Check sheet for the drawn part. Datum: minimum x, y, z corner. Units: mm. Round coordinates to 2 decimals unless told otherwise and drop trailing zeros. Write each loop counter-clockwise with the first axis right and the second up, starting at its lowest first coordinate (ties: lowest second). Pieces come first, ordered by that corner, then holes. Notation, with made-up numbers: (79, 30) - (84, 30) arc R20 cw to (84, 62) - close; hole circle Ø5 at (38, 71.25). An arc over 180 degrees is marked (long way). Answer as a JSON object with one key per item and string values.
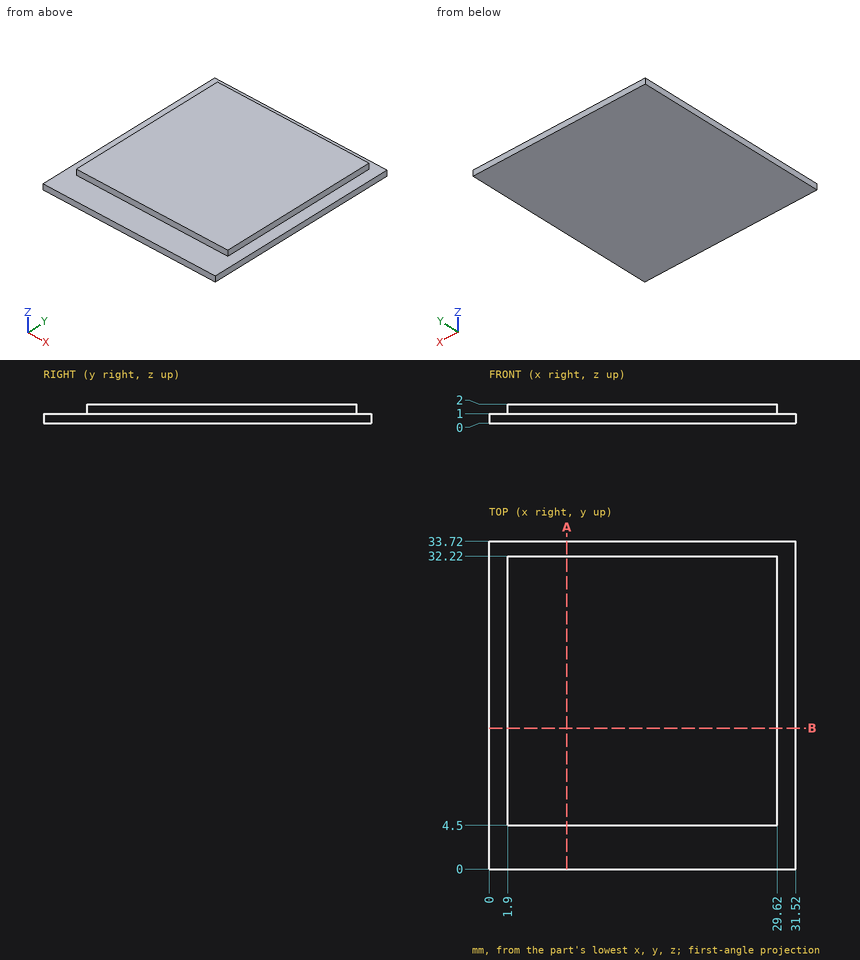
1. Material ranges on probe 1 along Y at (x, z) = (2.5, 1.1); probe 2 along Z at (x, y) = (22, 3.5); probe 3 along X at (y, z) = (10, 1.8), recorded low to high. Write a range as from..to.
Completed:
{"probe 1": "y = 4.5..32.22", "probe 2": "z = 0..1", "probe 3": "x = 1.9..29.62"}
2. Go/stop test with flat-tipped pins: pin 1 (10 mm diameter, centred on x = 26, y = 14, fed in from -Z); pin 2 (0.8 mm diameter, centred on y = 23.5, z = 1.5, fed in from -X); pin 3 (0.8 mm diameter, centred on x = 9, z = 1.5, fed in from -Y). Record where each tip stops, or that it passes through.
Completed:
{"pin 1": "stops at z = 0", "pin 2": "stops at x = 1.9", "pin 3": "stops at y = 4.5"}
3. Cross-section at B-B (y = 14.5). Record the boundary of the cut face in (x, z).
Completed:
{"outline": "(0, 0) - (31.52, 0) - (31.52, 1) - (29.62, 1) - (29.62, 2) - (1.9, 2) - (1.9, 1) - (0, 1) - close"}
4. Cross-section at A-A (x = 8). Record the boundary of the cut face in (y, z), plus the area to 3 significant figures.
Completed:
{"outline": "(0, 0) - (33.72, 0) - (33.72, 1) - (32.22, 1) - (32.22, 2) - (4.5, 2) - (4.5, 1) - (0, 1) - close", "area": "61.4 mm^2"}
